```python
from build123d import *

# Parameters (mm, degrees)
SKETCH_1_W           = 196
SKETCH_1_H           = 221
EXTRUDE_1_DEPTH      = 1.5
EXTRUDE_2_DEPTH      = 1.5
EXTRUDE_2_DEPTH_BACK = 10
SKETCH_4_W           = 159
SKETCH_4_H           = 3
EXTRUDE_3_DEPTH      = 1.5
SKETCH_8_W           = 159
SKETCH_8_H           = 0.5
SKETCH_8_W_2         = 149
SKETCH_8_H_2         = 75
SKETCH_8_H_3         = 17
CUT_EXTRUDE_5_DEPTH  = 41.5


with BuildPart() as part:
    # 草图1 → 凸台-拉伸1 (new body)
    with BuildSketch(Plane(origin=(0, 0, 0), x_dir=(1, 0, 0), z_dir=(0, 1, 0))):
        with Locations((98, 110.5)):
            Rectangle(SKETCH_1_W, SKETCH_1_H)
    extrude(amount=EXTRUDE_1_DEPTH)

    # 草图3 → 凸台-拉伸2 (add, two sides)
    with BuildSketch(Plane(origin=(0, 0, 0), x_dir=(1, 0, 0), z_dir=(0, 1, 0))) as extrude_2_sk:
        Polygon((3.5, 217.5), (27, 217.5), (27, 216.5), (186, 216.5), (186, 217.5), (192.5, 217.5), (192.5, 6), (192.5, 3.5), (172.5, 3.5), (172.5, 6), (190, 6), (190, 215), (6, 215), (6, 6), (23.5, 6), (23.5, 3.5), (3.5, 3.5), align=None)
    extrude(amount=EXTRUDE_2_DEPTH)
    extrude(extrude_2_sk.sketch, amount=-EXTRUDE_2_DEPTH_BACK)

    # 草图4 → 凸台-拉伸3 (add)
    with BuildSketch(Plane(origin=(0, 0, 0), x_dir=(1, 0, 0), z_dir=(0, 1, 0))):
        with Locations((106.5, 219.5)):
            Rectangle(SKETCH_4_W, SKETCH_4_H)
    extrude(amount=-EXTRUDE_3_DEPTH)

    # 草图8 → 切除-拉伸5 (cut)
    with BuildSketch(Plane(origin=(0, 1.5, 0), x_dir=(1, 0, 0), z_dir=(0, 1, 0))):
        Polygon((23.5, 0), (172.5, 0), (172.5, 20), (182.5, 20), (182.5, 80), (172.5, 80), (23.5, 80), (13.5, 80), (13.5, 20), (23.5, 20), align=None)
        with Locations((106.5, 217.75)):
            Rectangle(SKETCH_8_W, SKETCH_8_H)
        with Locations((98, 132.5)):
            Rectangle(SKETCH_8_W_2, SKETCH_8_H_2)
        with Locations((98, 194.5)):
            Rectangle(SKETCH_8_W_2, SKETCH_8_H_3)
    extrude(amount=-CUT_EXTRUDE_5_DEPTH, mode=Mode.SUBTRACT)


solid = part.part
```
Geometry check sheet. Reference: the model listing, model coordinates, mm. A direction names the side the tool comes from. Round coordinates to 2 decimals unless told otherwise and drop trailing zeros. Order: outer loops, then holes, each group sorted by start corner. A loop starts at its lowest first (then second) coordinate and runs counter-clockwise, first axis right, second up. Notation, with made-up numbers: M 72.25,72 L 121.25,72 A27 cw 121.25,91 Z; hole C 81,89.25 d5. An arc over 180 degrees is marked long. Write item = value, one per line.
Q1. Section check C-C (y = -6.25). Enter the section's corners in (x, z), plus the area to 3 significant figures.
Answer block:
outline = M 3.5,-217.5 L 27,-217.5 L 27,-216.5 L 186,-216.5 L 186,-217.5 L 192.5,-217.5 L 192.5,-3.5 L 172.5,-3.5 L 172.5,-6 L 190,-6 L 190,-215 L 6,-215 L 6,-6 L 23.5,-6 L 23.5,-3.5 L 3.5,-3.5 Z
area = 1,460 mm^2
Q2. Section check B-B (x = 143). Enter the section's corners in (y, z).
Answer block:
outline = M -10,-216.5 L 0,-216.5 L 0,-217.5 L 1.5,-217.5 L 1.5,-203 L 0,-203 L 0,-215 L -10,-215 Z; M -1.5,-221 L 1.5,-221 L 1.5,-218 L -1.5,-218 Z; M 0,-186 L 1.5,-186 L 1.5,-170 L 0,-170 Z; M 0,-95 L 1.5,-95 L 1.5,-80 L 0,-80 Z
Q3. Set-up check for faces 5 (the flat face through (172.5, 0.5, -7.7)), 6 (the flat face through (192.5, -5, -109)), 7 (the flat face through (3.5, -5, -109)), 8 (the flat face through (190, -5, -109)): record each of +Z, -Z, +X, -X, +Y, -Y from which the full face is reachable in a straight line by a thin tool's end or side.
Answer block:
face_5 = +Z, +Y, -Y
face_6 = +Z, -Z, +X, -Y
face_7 = +Z, -Z, -X, -Y
face_8 = -Y
Q4. Section check A-A (z = -103). Enter the section's corners in (x, y).
Answer block:
outline = M 0,0 L 3.5,0 L 3.5,-10 L 6,-10 L 6,0 L 23.5,0 L 23.5,1.5 L 0,1.5 Z; M 172.5,0 L 190,0 L 190,-10 L 192.5,-10 L 192.5,0 L 196,0 L 196,1.5 L 172.5,1.5 Z
Q5. Scan lines: line 1 (Z direction, x = 98, y = 1); line 2 (X direction, y = -0.5, z = -59); line 3 (X direction, y = 1, z = -148). Record each from-to range of solid material in increasing order.
Answer block:
line_1 = -221 to -218, -217.5 to -203, -186 to -170, -95 to -80
line_2 = 3.5 to 6, 190 to 192.5
line_3 = 0 to 23.5, 172.5 to 196
Q6. Release check for a two-part mould opening along Z. For faces 1 (the flat face through (1, 0, -111)), 2 (the flat face through (6, -5, -112)), 3 (the flat face through (14, -5, -3.5)), 4 (the flat face through (97, 0, -182)) record: released by +Z, released by -Z, zero draft, split by the parting line, or undercut.
Answer block:
face_1 = zero draft
face_2 = undercut
face_3 = released by +Z
face_4 = undercut
Q7. Depth check by flat-ended pin: pin 1 Ø2 at (x, y) = (169, -7.5) entering from -Z; pin 2 Ø3 at (y, z) = (-3.5, -128) entering from -X; pin 3 Ø12 at (x, z) = (25.5, -137) entering from -Y. Enter the tip coordinate at first touch or a pass-through.
Answer block:
pin_1 = -216.5
pin_2 = 3.5
pin_3 = 0
